Could you check a few things on this model? Use its own coordinates, in mm. A direction names the side the tool comes from. Give positions to 0.01 mm unless a question says otherwise; leave off trailing zeros. Write each loop counter-clockwise with the first axis right and the second up, starting at its lowest first coordinate (ties: lowest second). Pieces come first, ordered by that corner, then holes. Notation, with made-up numbers: M 51,-20.75 L 56,-20.75 A14 cw 56,-4.75 Z; hole C 76.25,66 d3. An arc over 180 degrees is marked long. Use one line per item in the form item = value.
from build123d import *

# Parameters (mm, degrees)
F0_R     = 3.96875
F1_DEPTH = 200.914
F2_W     = 4.572
F2_H     = 0.24765


with BuildPart() as f1:
    # F0 (on Right) → F1 (new body)
    with BuildSketch(Plane.YZ):
        Circle(F0_R)
    extrude(amount=F1_DEPTH)

    # F2 (on Front) → F3 (revolve, cut)
    with BuildSketch(Plane.XZ):
        with Locations((185.166, 3.844925)):
            Rectangle(F2_W, F2_H)
        with Locations((92.964, 3.844925)):
            Rectangle(F2_W, F2_H)
        with Locations((4.826, 3.844925)):
            Rectangle(F2_W, F2_H)
    revolve(axis=Axis((98.498309, 0, 0), (1, 0, 0)), mode=Mode.SUBTRACT)


solid = f1.part
1) Thinking about a two-plate mould opening in X: for faces 1 (the cylindrical face through (48.31, 3.785, 1.192)), 2 (the flat face through (200.914, 0, 0)), 3 (the cylindrical face through (185.2, -1.12, 3.55)), which applies, released by +X, released by -X, zero draft, split by the parting line, or undercut?
Checked values:
face_1 = zero draft
face_2 = released by +X
face_3 = undercut
2) If I drill on L1, parallel to X at y = 2.25, z = 3; L2, parallel to Y at x = 126.5, z = -0.25; L3, parallel to Y at x = 123, z = 0.5, over which ranges is the centre line in solid material (lowest first)?
Checked values:
L1 = 0 to 2.54, 7.11 to 90.68, 95.25 to 182.88, 187.45 to 200.91
L2 = -3.96 to 3.96
L3 = -3.94 to 3.94
3) For faces 4 (the flat face through (0, 0, 0)), 5 (the cylindrical face through (93, -1.12, 3.55)), which set-ups out of +Z, -Z, +X, -X, +Y, -Y let a thin tool reach every point of the face, with its end or its side?
Checked values:
face_4 = +Z, -Z, -X, +Y, -Y
face_5 = none
4) I want a section at C-C, the plane z = -2. Please give me the cut outline in (x, y), plus the area to 3 significant figures.
Checked values:
outline = M 0,-3.43 L 2.54,-3.43 L 2.54,-3.14 L 7.11,-3.14 L 7.11,-3.43 L 90.68,-3.43 L 90.68,-3.14 L 95.25,-3.14 L 95.25,-3.43 L 182.88,-3.43 L 182.88,-3.14 L 187.45,-3.14 L 187.45,-3.43 L 200.91,-3.43 L 200.91,3.43 L 187.45,3.43 L 187.45,3.14 L 182.88,3.14 L 182.88,3.43 L 95.25,3.43 L 95.25,3.14 L 90.68,3.14 L 90.68,3.43 L 7.11,3.43 L 7.11,3.14 L 2.54,3.14 L 2.54,3.43 L 0,3.43 Z
area = 1,370 mm2
5) I want a section at B-B, the plane x = 157.5. Please give me the cut outline in (y, z), plus the area to 3 significant figures.
Checked values:
outline = C 0,0 d7.94
area = 49.5 mm2
6) For pin 1 Ø4 at (y, z) = (1, -1) entering from -X; pin 2 Ø3 at (x, z) = (43, -3) entering from -Y, each with a flat end and sliding along its axis, tell me the tip position at first contact or that it passes through.
Checked values:
pin_1 = 0
pin_2 = -3.67
7) I want a section at A-A, the plane y = 2.25. Please give me the cut outline in (x, z).
Checked values:
outline = M 0,-3.27 L 2.54,-3.27 L 2.54,-2.96 L 7.11,-2.96 L 7.11,-3.27 L 90.68,-3.27 L 90.68,-2.96 L 95.25,-2.96 L 95.25,-3.27 L 182.88,-3.27 L 182.88,-2.96 L 187.45,-2.96 L 187.45,-3.27 L 200.91,-3.27 L 200.91,3.27 L 187.45,3.27 L 187.45,2.96 L 182.88,2.96 L 182.88,3.27 L 95.25,3.27 L 95.25,2.96 L 90.68,2.96 L 90.68,3.27 L 7.11,3.27 L 7.11,2.96 L 2.54,2.96 L 2.54,3.27 L 0,3.27 Z
